```python
from build123d import *

# Parameters (mm, degrees)
ESQUISSE1_R             = 16
BOSS_EXTRU_1_DEPTH      = 1
ESQUISSE2_R             = 12.5
BOSS_EXTRU_2_DEPTH      = 7
ESQUISSE3_R             = 16
BOSS_EXTRU_3_DEPTH      = 1
ESQUISSE4_R             = 8
BOSS_EXTRU_4_DEPTH      = 5
ESQUISSE5_R             = 2.5
ENL_V_MAT_EXTRU_1_DEPTH = 15


with BuildPart() as part:
    # Esquisse1 → Boss.-Extru.1 (new body)
    with BuildSketch(Plane.XY):
        Circle(ESQUISSE1_R)
    extrude(amount=BOSS_EXTRU_1_DEPTH)

    # Esquisse2 → Boss.-Extru.2 (add)
    with BuildSketch(Plane.XY.offset(1)):
        Circle(ESQUISSE2_R)
    extrude(amount=BOSS_EXTRU_2_DEPTH)

    # Esquisse3 → Boss.-Extru.3 (add)
    with BuildSketch(Plane.XY.offset(8)):
        Circle(ESQUISSE3_R)
    extrude(amount=BOSS_EXTRU_3_DEPTH)

    # Esquisse4 → Boss.-Extru.4 (add)
    with BuildSketch(Plane.XY.offset(9)):
        Circle(ESQUISSE4_R)
    extrude(amount=BOSS_EXTRU_4_DEPTH)

    # Esquisse5 → Enlèv. mat.-Extru.1 (cut, through all)
    with BuildSketch(Plane.XY.offset(14)):
        Circle(ESQUISSE5_R)
    extrude(amount=-ENL_V_MAT_EXTRU_1_DEPTH, mode=Mode.SUBTRACT)

    # Esquisse7 → Dégagement M31 (revolve, cut)
    with BuildSketch(Plane(origin=(-8, 0, 11.497538613), x_dir=(0, 0, 1), z_dir=(0, 1, 0))):
        Polygon((0, 0), (0, 8), (1.6, 8), (1.6, 0.025), (1.625, 0), align=None)
    revolve(axis=Axis((-14.35, 0, 11.497538613), (1, 0, 0)), mode=Mode.SUBTRACT)


solid = part.part
```
The listing builds one solid part. Answer for the finished solid, in the listing's coordinates (mm). A direction names the side the tool comes from. Coordinates: 2 decimals unless noted, no trailing zeros. Write each loop counter-clockwise with the first axis right and the second up, starting at its lowest first coordinate (ties: lowest second). Pieces come first, ordered by that corner, then holes. Notation, with made-up numbers: (4.5, 75.5) - (33.5, 75.5) arc R10 ccw to (33.5, 91.5) - close; hole circle Ø8 at (-38.75, -28). An arc over 180 degrees is marked (long way). One line per item, written item: value.
1) A tool of negligible diameter and unlimited length cuts with its end or side. For faces 4 (the cylindrical face through (-3.47, -15.62, 8.49)), 5 (the flat face through (-3.8, 7.3, 9)), 6 (the cylindrical face through (-4.99, -1.586, 11.289)), 7 (the flat face through (-10, -8, 1)), from which of +Z, -Z, +X, -X, +Y, -Y can it reach the whole face along a straight path? Write none if from no direction.
Geometry check:
face 4: +Z, -Z
face 5: +Z
face 6: -X
face 7: none
2) Find section C-C (y = -14). Give the vertices of the cut face in (x, z).
Geometry check:
outline: (-7.75, 0) - (7.75, 0) - (7.75, 1) - (-7.75, 1) - close; (-7.75, 8) - (7.75, 8) - (7.75, 9) - (-7.75, 9) - close
3) Find section B-B (y = 0). Give the vertices of the cut face in (x, z) (3 decimals).
Geometry check:
outline: (-16, 0) - (-2.5, 0) - (-2.5, 9.898) - (-7.975, 9.898) - (-8, 9.873) - (-8, 9) - (-16, 9) - (-16, 8) - (-12.5, 8) - (-12.5, 1) - (-16, 1) - close; (-8, 13.123) - (-7.975, 13.098) - (-2.5, 13.098) - (-2.5, 14) - (-8, 14) - close; (2.5, 0) - (16, 0) - (16, 1) - (12.5, 1) - (12.5, 8) - (16, 8) - (16, 9) - (8, 9) - (8, 14) - (2.5, 14) - close
4) Find section A-A (x = 0). Give the vertices of the cut face in (y, z).
Geometry check:
outline: (-16, 0) - (-2.5, 0) - (-2.5, 14) - (-8, 14) - (-8, 9) - (-16, 9) - (-16, 8) - (-12.5, 8) - (-12.5, 1) - (-16, 1) - close; (2.5, 0) - (16, 0) - (16, 1) - (12.5, 1) - (12.5, 8) - (16, 8) - (16, 9) - (8, 9) - (8, 14) - (2.5, 14) - close
5) Consider line 1 along Y through (x, z) = (0, 6.25); line 2 along Z through (x, y) = (-2, 13); line 3 along X through (y, z) = (0, 9.5). Determine where each line is inside the solid, lowest interval first. Write a range as from..to.
Geometry check:
line 1: y = -12.5..-2.5, 2.5..12.5
line 2: z = 0..1, 8..9
line 3: x = -8..-2.5, 2.5..8
6) Each of these flat-tipped pins is pushed along its axis until it touches: pin 1 Ø3 at (x, z) = (1.5, 5) entering from -Y; pin 2 Ø4 at (y, z) = (7, 10) entering from +X; pin 3 Ø3 at (y, z) = (-2.5, 11.5) entering from -X. Where does it stop, or does it pass through?
Geometry check:
pin 1: stops at y = -12.5
pin 2: stops at x = 15.11
pin 3: stops at x = -7.89
7) Find section D-D (x = -4). Give the vertices of the cut face in (y, z), and give its area (3 significant figures).
Geometry check:
outline: (-15.49, 0) - (15.49, 0) - (15.49, 1) - (11.84, 1) - (11.84, 8) - (15.49, 8) - (15.49, 9) - (6.93, 9) - (6.93, 14) - (-6.93, 14) - (-6.93, 9) - (-15.49, 9) - (-15.49, 8) - (-11.84, 8) - (-11.84, 1) - (-15.49, 1) - close; hole circle Ø3.2 at (0, 11.5)
area: 289 mm2
8) For a pull along Y with two mould halves and no side action, classify faces 1 (the cylindrical face through (2.385, 0.751, 7.098)), 2 (the cylindrical face through (7.39, -3.06, 11.46)), 3 (the flat face through (-10, -8, 8)) as pulls with the +Y half, pulls with the -Y half, needs draft (parallel to the pull), parting line crosses it, or undercut.
Geometry check:
face 1: undercut
face 2: parting line crosses it
face 3: needs draft
